Can you work these out from the model? Positions are in its coordinate system, mm. A direction names the side the tool comes from. Round coordinates to 2 decimals unless told otherwise and drop trailing zeros. Loops run counter-clockwise (first coordinate to the right, second up) from the corner with the lowest first, then second, coordinate; pieces in that order, holes last. Notation, with made-up numbers: (-13, 36) - (13, 36) arc R23 ccw to (13, 62) - close; hole circle Ø1 at (37, 63). An arc over 180 degrees is marked (long way). Answer as CSV lines item,"result".
Autodesk Fusion 360 part; units mm, degrees
sketch "Sketch1" plane through (0, 0, 0) normal (0, 0, 1) x (1, 0, 0)
  circle A0 centre (0, 0) radius 2
  dimension "d1" = 4
extrude "Extrude1" add sketch "Sketch1" along normal blind 6.2
sketch "Sketch2" plane through (0, 0, 6.2) normal (0, 0, 1) x (-1, 0, 0)
  circle A0 centre (0, 0) radius 2
  circle A1 centre (0, 0) radius 0.875
  dimension "d4" = 1.75
extrude "Extrude2" add sketch "Sketch2" along normal blind 1.5 contours A1
chamfer "Chamfer2" distance 1.1 angle 45 1 edges at (-1.8647, -0.7232, 0)
extrude "Extrude4" add 1 faces at (0.4737, -0.323, 0) along direction (0, 0, -1) blind 1
Q1. I'm going to push flat-ended pins straight in: pin 1 Ø1 at (y, z) = (1, 2.5) entering from +X; pin 2 Ø2 at (x, y) = (0, -1) entering from +Z. Where does each tip first touch, or does it pass through?
Checks:
pin 1,"x = 1.94"
pin 2,"z = 7.7"
Q2. Imagine slicing it at A-A (x = 0). Write out the boundary of the cut face in (y, z) (3 decimals).
Checks:
outline,"(-2, 1.1) - (-0.9, 0) - (-0.9, -1) - (0.9, -1) - (0.9, 0) - (2, 1.1) - (2, 6.2) - (0.875, 6.2) - (0.875, 7.7) - (-0.875, 7.7) - (-0.875, 6.2) - (-2, 6.2) - close"
Q3. On a 3-axis mill with a long thin cutter (end or side, diameter ignored), from which of +Z, -Z, +X, -X, +Y, -Y can I reach the whole of each face in a straight line? I mean faces 1 (the flat face through (0, 0, 7.7)), 2 (the flat face through (0.9, 0.5, 6.2)), 3 (the cylindrical face through (0.86, 0.27, -0.49)). Say none if no direction works.
Checks:
face 1,"+Z, +X, -X, +Y, -Y"
face 2,"+Z"
face 3,"-Z"
Q4. If I drill on line 1 along X through (y, z) = (-0.1, 2.25); line 2 along Z through (x, y) = (0.5, 1.7); line 3 along X through (y, z) = (-0.9, 2.5), over which ranges is the centre line in solid material (lowest first)? Write a range as [from, to].
Checks:
line 1,"[-2, 2]"
line 2,"[0.87, 6.2]"
line 3,"[-1.79, 1.79]"
Q5. Imagine slicing it at C-C (z = 3.75). Write out the boundary of the cut face in (x, y).
Checks:
outline,"circle Ø4 at (0, 0)"
